from build123d import *

# Parameters (mm, degrees)
F0_W     = 202.4
F0_H     = 381
F1_DEPTH = 3
F2_D     = 6.6


with BuildPart() as f1:
    # F0 (on Front) → F1 (new body)
    with BuildSketch(Plane.XZ):
        with Locations((-61.9627135719, -1.6996394843)):
            Rectangle(F0_W, F0_H)
    extrude(amount=F1_DEPTH)

    # F2 (through all)
    with Locations(Plane(origin=(0, 0, 0), x_dir=(1, 0, 0), z_dir=(0, 1, 0))):
        with Locations((-150.6627135719, -163.4003605157), (-150.6627135719, -11.0003605157), (-150.6627135719, 141.3996394843), (26.7372864281, 141.3996394843), (26.7372864281, -11.0003605157), (26.7372864281, -163.4003605157)):
            Hole(F2_D / 2)


solid = f1.part
Can you work these out from the model? Positions are in its coordinate system, mm. Coordinates: 2 decimals unless noted, no trailing zeros.
Q1. If we mould it in two halves opening along Z, with no side actions, what happens to faces 1 (the face through (-153.711, -1.521, 164.664)), 2 (the face through (-63, 0, 1)), 3 (the face through (30.034, -1.521, 10.855))? For each: +Z half, -Z half, draft (parallel to the pull), parting line (faces both ways), or undercut.
Results found:
face 1: undercut
face 2: draft
face 3: undercut
Q2. For P1, Ø6, axis at x = 26.74, z = -141.4, coming from the +Y side, with a flat end and sliding along its axis, tell me the tip position at first contact or that it passes through.
Results found:
P1: passes through
Q3. Please list where this line runs through material, in increasing order: L1, parallel to Z at x = 24.5, y = -0.55.
Results found:
L1: z = -192.2 to -143.83, -138.97 to 8.57, 13.43 to 160.97, 165.83 to 188.8
